from build123d import *

# Parameters (mm, degrees)
F1_DEPTH = 170
F5_DEPTH = 9


with BuildPart() as f1:
    # F0 (on Front) → F1 (new body)
    with BuildSketch(Plane.XZ):
        Polygon((4.999971, -0.017115), (2.514808, 4.321544), (-2.485163, 4.338659), (-4.999971, 0.017115), (-2.514808, -4.321544), (2.485163, -4.338659), align=None)
    extrude(amount=F1_DEPTH)

    # F2 (on Top) → F3 (revolve)
    with BuildSketch(Plane.XY):
        Polygon((-4.33, 0), (0, 0), (0, 12), align=None)
    revolve(axis=Axis((0, 6, 0), (0, 1, 0)))

    # F4 (on face) → F5 (join)
    with BuildSketch(Plane.XZ.offset(170)):
        with BuildLine():
            ThreePointArc((3.893099, -1.919207), (4.227139, -0.985328), (4.340458, 0))
            ThreePointArc((4.340458, 0), (4.230487, 0.970853), (3.906147, 1.89251))
            Line((3.906147, 1.89251), (3.608632, 2.411919))
            ThreePointArc((3.608632, 2.411919), (2.183083, 3.751496), (0.314112, 4.329077))
            Line((0.314112, 4.329077), (-0.284467, 4.331126))
            ThreePointArc((-0.284467, 4.331126), (-2.157349, 3.766354), (-3.592035, 2.436567))
            Line((-3.592035, 2.436567), (-3.893099, 1.919207))
            ThreePointArc((-3.893099, 1.919207), (-4.340433, 0.014858), (-3.906147, -1.89251))
            Line((-3.906147, -1.89251), (-3.608632, -2.411919))
            ThreePointArc((-3.608632, -2.411919), (-2.183083, -3.751496), (-0.314112, -4.329077))
            Line((-0.314112, -4.329077), (0.284467, -4.331126))
            ThreePointArc((0.284467, -4.331126), (2.157349, -3.766354), (3.592035, -2.436567))
            Line((3.592035, -2.436567), (3.893099, -1.919207))
        make_face()
    extrude(amount=F5_DEPTH)


solid = f1.part
Source: CAD feature listing. Evaluate the final solid. Frame: model axes, mm. A direction names the side the tool comes from. Coordinates: 2 decimals unless noted, no trailing zeros. Order: outer loops, then holes, each group sorted by start corner. A loop starts at its lowest first (then second) coordinate and runs counter-clockwise, first axis right, second up.
Item 1: Set-up query: faces 1 (the face through (-4.34, -174.44, 0.04)), 2 (the face through (-2.1, -174.4, 3.8)), 3 (the face through (-2.207, -174.437, -3.738)), 4 (the face through (2.207, -174.437, 3.738)), 5 (the face through (2.1, -174.4, -3.8)). Return all of +Z, -Z, +X, -X, +Y, -Y with unobstructed straight access to the full face (end or side cutting, diameter ignored); none if empty.
Output values:
face 1: -X, -Y
face 2: +Z, -X, -Y
face 3: -Z, -X, -Y
face 4: +Z, +X, -Y
face 5: -Z, +X, -Y
Item 2: First-contact query: P1, Ø2, axis at x = -1.5, y = -66.5, coming from the -Z side; P2, Ø1.5, axis at y = -55.5, z = 1.5, coming from the -X side; P3, Ø1, axis at x = 4, z = 3, coming from the +Y side. Flat tips, straight axial feed; report the tip coordinate or a pass-through.
Output values:
P1: stops at z = -4.33
P2: stops at x = -4.57
P3: passes through
Item 3: Material intervals for line 1 (X direction, y = -22, z = 2.5); line 2 (Z direction, x = -1.75, y = -33.5); line 3 (X direction, y = -61, z = 0), sorted ascending.
Output values:
line 1: x = -3.56 to 3.56
line 2: z = -4.32 to 4.34
line 3: x = -4.99 to 4.99
Item 4: Cut plane A-A (y = -145). Return loops of the section in (x, z), plus the area to 3 significant figures.
Output values:
outline: (-5, 0.02) - (-2.51, -4.32) - (2.49, -4.34) - (5, -0.02) - (2.51, 4.32) - (-2.49, 4.34) - close
area: 65.0 mm2
